Autodesk Inventor part; units mm, degrees
ref_plane "YZ Plane" through (0, 0, 0) normal (1, 0, 0) x (0, 1, 0)
ref_plane "XZ Plane" through (0, 0, 0) normal (0, 1, 0) x (-1, 0, 0)
ref_plane "XY Plane" through (0, 0, 0) normal (0, 0, 1) x (1, 0, 0)
ref_plane "Arbeitsebene1" through (0, 0, 0) normal (0, 0, 1) x (1, 0, 0)
sketch "Skizze1" plane through (0, 0, 0) normal (0, 0, 1) x (1, 0, 0)
  line L0 (9.1071, 105.908) -> (0.6071, 100.2819) construction
  arc A0 (9.1071, 105.908) -> (9.6, 106.8252) centre (8.5, 106.8252) ccw construction
  line L1 (9.6, 121.5) -> (9.6, 106.8252) construction
  arc A1 (9.6, 121.5) -> (8.5, 122.6) centre (8.5, 121.5) ccw construction
  line L2 (-8.5, 122.6) -> (8.5, 122.6) construction
  arc A2 (-8.5, 122.6) -> (-9.6, 121.5) centre (-8.5, 121.5) ccw construction
  line L3 (-9.6, 106.8252) -> (-9.6, 121.5) construction
  arc A3 (-9.6, 106.8252) -> (-9.1071, 105.908) centre (-8.5, 106.8252) ccw construction
  line L4 (-0.6071, 100.2819) -> (-9.1071, 105.908) construction
  arc A4 (-0.6071, 100.2819) -> (0.6071, 100.2819) centre (0, 101.1992) ccw construction
  circle A5 centre (5.6569, 118.6569) radius 1.6 construction
  circle A6 centre (5.6569, 107.3431) radius 1.6 construction
  circle A7 centre (-5.6569, 107.3431) radius 1.6 construction
  circle A8 centre (-5.6569, 118.6569) radius 1.6 construction
  circle A9 centre (0, 113) radius 3 construction
  arc A10 (-8.5, 122.4) -> (-9.4, 121.5) centre (-8.5, 121.5) ccw
  line L5 (-8.5, 122.4) -> (8.5, 122.4)
  arc A11 (9.4, 121.5) -> (8.5, 122.4) centre (8.5, 121.5) ccw
  line L6 (9.4, 121.5) -> (9.4, 106.8252)
  arc A12 (8.9967, 106.0747) -> (9.4, 106.8252) centre (8.5, 106.8252) ccw
  line L7 (8.9967, 106.0747) -> (0.4967, 100.4487)
  arc A13 (-0.4967, 100.4487) -> (0.4967, 100.4487) centre (0, 101.1992) ccw
  line L8 (-0.4967, 100.4487) -> (-8.9967, 106.0747)
  arc A14 (-9.4, 106.8252) -> (-8.9967, 106.0747) centre (-8.5, 106.8252) ccw
  line L9 (-9.4, 106.8252) -> (-9.4, 121.5)
  point P0 (0, 0)
  dimension "d2" = 0
  dimension "d0" = 0.2
extrude "Extrusion1" add sketch "Skizze1" along normal blind 1
properties part number "Cover_Robot_Motor_Shoulder"
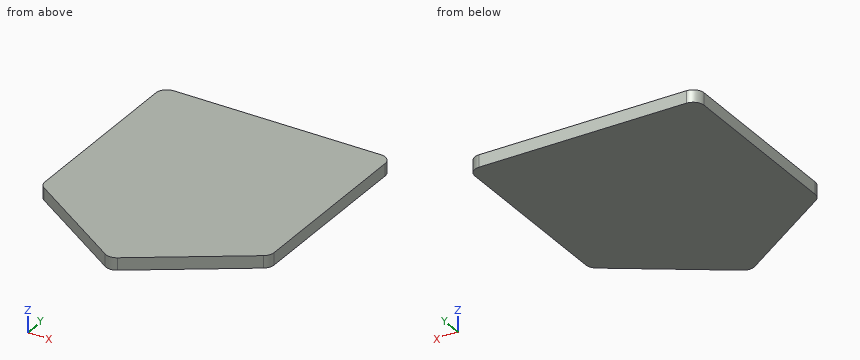
Geometry check sheet. Reference: the model listing, model coordinates, mm. Coordinates: 2 decimals unless noted, no trailing zeros. Order: outer loops, then holes, each group sorted by start corner. A loop starts at its lowest first (then second) coordinate and runs counter-clockwise, first axis right, second up. Notation, with made-up numbers: M -40,22.25 L 13,22.25 A21 ccw 13,26.25 Z; hole C 25.5,73.5 d7. An arc over 180 degrees is marked long. Answer as a JSON object with one key per item and string values.
Q1. Cross-section at C-C on y = 105. Record the cut outline in (x, z).
Results are:
{"outline": "M -7.37,0 L 7.37,0 L 7.37,1 L -7.37,1 Z"}
Q2. Scan lines: line 1 (Y direction, x = 3, z = 0.25); line 2 (Y direction, x = -3.75, z = 0.5); line 3 (X direction, y = 104, z = 0.25). Record each from-to range of solid material in increasing order.
Results are:
{"line 1": "y = 102.11 to 122.4", "line 2": "y = 102.6 to 122.4", "line 3": "x = -5.86 to 5.86"}
Q3. Cross-section at B-B on x = -7.25. Record the cut outline in (y, z).
Results are:
{"outline": "M 104.92,0 L 122.4,0 L 122.4,1 L 104.92,1 Z"}
Q4. Cross-section at A-A on z = 0.3. Record the cut outline in (x, y).
Results are:
{"outline": "M -9.4,106.83 A0.9 ccw -9,106.07 L -0.5,100.45 A0.9 ccw 0.5,100.45 L 9,106.07 A0.9 ccw 9.4,106.83 L 9.4,121.5 A0.9 ccw 8.5,122.4 L -8.5,122.4 A0.9 ccw -9.4,121.5 Z"}
